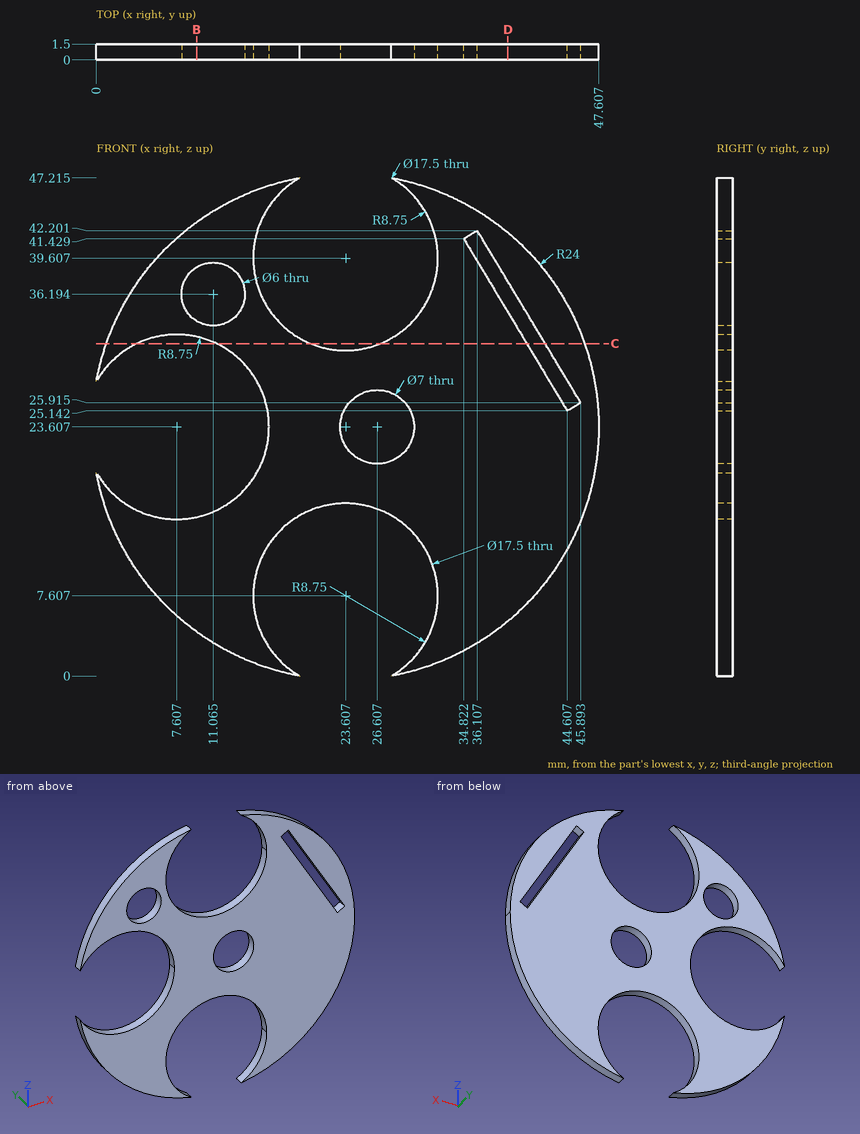
Here's the drawing with two shaded views (mm, measured from the low corner). I have some questions. Give positions to 0.01 mm unless a question says otherwise; leave off trailing zeros. Order: outer loops, then holes, each group sorted by start corner. A loop starts at its lowest first (then second) coordinate and runs counter-clockwise, first axis right, second up.
Q1. Suppose I cut it at C-C, the plane z = 31.5. Write out the boundary of the cut face in (x, y) (1 decimal).
Q2. Suppose I cut it at D-D, the plane x = 39. Write out the boundary of the cut face in (y, z) (1 decimal).
Q3. I'm going to push a flat-ended pin straight in: P1, Ø5.5, axis at x = 11.06, z = 36.19, coming from the +Y side. Where does the tip first touch, or does it pass through?
Q4. Suppose I cut it at B-B, the plane x = 9.5. Count the separate pieces of the cut face and the enclosed holes in it.
Q5. If I drill on line 1 along Z through (x, y) = (12.5, 0.1) (1 decimal); line 2 along Z through (x, y) = (31, 0.6) (1 decimal); line 3 along X through (y, z) = (1.2, 12) (1 decimal), over which ranges is the centre line in solid material (lowest first)?
Solution:
1. outline: (0.9, 0) - (3.8, 0) - (3.8, 1.5) - (0.9, 1.5) - close; (11.4, 0) - (20.3, 0) - (20.3, 1.5) - (11.4, 1.5) - close; (26.9, 0) - (40.8, 0) - (40.8, 1.5) - (26.9, 1.5) - close; (42.5, 0) - (46.3, 0) - (46.3, 1.5) - (42.5, 1.5) - close
2. outline: (0, 5.2) - (1.5, 5.2) - (1.5, 34.5) - (0, 34.5) - close; (0, 37.4) - (1.5, 37.4) - (1.5, 42) - (0, 42) - close
3. P1: passes through
4. separate pieces: 3
4. enclosed holes: 0
5. line 1: z = 2.3 to 16.4, 30.9 to 33.6, 38.8 to 44.9
5. line 2: z = 0.8 to 2.9, 12.3 to 34.9, 44.3 to 46.4
5. line 3: x = 2.6 to 16, 31.2 to 44.6
